from build123d import *
from OCP.BRepFilletAPI import BRepFilletAPI_MakeChamfer

# Parameters (mm, degrees)
SKETCH2_R               = 67.5
SKETCH2_W               = 66.7
SKETCH2_H               = 90
BOSS_EXTRUDE1_DEPTH     = 15
SKETCH7_W               = 14
SKETCH7_H               = 11.1
CUT_EXTRUDE1_DEPTH      = 135.058839694
CUT_EXTRUDE1_DEPTH_BACK = 135.058839694
SKETCH8_R               = 9.5
FILLET1_R               = 20
SKETCH9_R               = 2.1
CUT_EXTRUDE2_DEPTH      = 97.630740606
CHAMFER1_SIZE           = 1.5
CHAMFER1_SIZE2          = 0.866025404
SKETCH10_R              = 4.1
CUT_EXTRUDE3_DEPTH      = 97.630740606
CUT_EXTRUDE4_DEPTH      = 97.630740606
SKETCH12_W              = 10
SKETCH12_H              = 6
CUT_EXTRUDE5_DEPTH      = 97.630740606
CHAMFER2_START          = -1
CHAMFER2_DEPTH          = 16
CUT_EXTRUDE6_DEPTH      = 97.630740606


with BuildPart() as part:
    # Sketch2 → Boss-Extrude1 (new body)
    with BuildSketch(Plane(origin=(0, 0, 0), x_dir=(1, 0, 0), z_dir=(0, 1, 0))):
        with Locations(Location((0, 0, 0), (0, 0, 270))):
            Circle(SKETCH2_R)
        Rectangle(SKETCH2_W, SKETCH2_H, mode=Mode.SUBTRACT)
    extrude(amount=BOSS_EXTRUDE1_DEPTH)

    # Sketch7 → Cut-Revolve2 (revolve, cut)
    with BuildSketch(Plane(origin=(0, 15, 0), x_dir=(1, 0, 0), z_dir=(0, 1, 0))):
        with Locations((-40.35, 5.55)):
            Rectangle(SKETCH7_W, SKETCH7_H)
        with Locations((40.35, 5.55)):
            Rectangle(SKETCH7_W, SKETCH7_H)
    revolve(axis=Axis((67.5, 15, 0), (-1, 0, 0)), mode=Mode.SUBTRACT)

    # Sketch8 → Cut-Extrude1 (cut, two sides: drawn at the far end of the back side and taken through both)
    with BuildSketch(Plane.ZY.offset(-47.35).offset(-CUT_EXTRUDE1_DEPTH_BACK)):
        with Locations((0, 15)):
            Circle(SKETCH8_R)
    extrude(amount=CUT_EXTRUDE1_DEPTH + CUT_EXTRUDE1_DEPTH_BACK, mode=Mode.SUBTRACT)

    # Fillet1
    fillet1_edges = [part.edges().sort_by_distance(p)[0] for p in [
        (-33.35, 7.5, -45),
        (-33.35, 7.5, 45),
        (33.35, 7.5, 45),
        (33.35, 7.5, -45),
    ]]
    fillet(fillet1_edges, radius=FILLET1_R)

    # Sketch9 → Cut-Extrude2 (cut, through all)
    with BuildSketch(Plane(origin=(0, 15, 0), x_dir=(1, 0, 0), z_dir=(0, 1, 0))):
        with Locations(Location((-37.629775444, 17.5, 0), (0, 0, 270))):
            Circle(SKETCH9_R)
        with Locations(Location((37.629775444, 17.5, 0), (0, 0, 270))):
            Circle(SKETCH9_R)
        with Locations(Location((37.629775444, -17.5, 0), (0, 0, 270))):
            Circle(SKETCH9_R)
        with Locations(Location((-37.629775444, -17.5, 0), (0, 0, 270))):
            Circle(SKETCH9_R)
        with Locations(Location((-20, 51.23475383, 0), (0, 0, 270))):
            Circle(SKETCH9_R)
        with Locations(Location((20, 51.23475383, 0), (0, 0, 270))):
            Circle(SKETCH9_R)
        with Locations(Location((20, -51.23475383, 0), (0, 0, 270))):
            Circle(SKETCH9_R)
        with Locations(Location((-20, -51.23475383, 0), (0, 0, 270))):
            Circle(SKETCH9_R)
        with Locations(Location((0, -55, 0), (0, 0, 270))):
            Circle(SKETCH9_R)
        with Locations(Location((0, 58.5, 0), (0, 0, 270))):
            Circle(SKETCH9_R)
        with Locations(Location((-46, 17.5, 0), (0, 0, 270))):
            Circle(SKETCH9_R)
        with Locations(Location((46, 17.5, 0), (0, 0, 270))):
            Circle(SKETCH9_R)
        with Locations(Location((46, -17.5, 0), (0, 0, 270))):
            Circle(SKETCH9_R)
        with Locations(Location((-46, -17.5, 0), (0, 0, 270))):
            Circle(SKETCH9_R)
    extrude(amount=-CUT_EXTRUDE2_DEPTH, mode=Mode.SUBTRACT)

    # Chamfer1: one chamfer whose edges measure the first distance from different faces: ONE call of the kernel's chamfer builder (chamfer() names one face for all edges)
    chamfer1_edges_1 = [part.edges().sort_by_distance(p)[0] for p in [
        (-33.35, 3.9, 0),
    ]]
    chamfer1_side_1 = [part.faces().sort_by_distance(p)[0] for p in [
        (-33.35, 0.522015325, 0),
    ]]
    chamfer1_edges_2 = [part.edges().sort_by_distance(p)[0] for p in [
        (33.35, 3.9, 0),
    ]]
    chamfer1_side_2 = [part.faces().sort_by_distance(p)[0] for p in [
        (33.35, 0.522015325, 0),
    ]]
    chamfer1 = BRepFilletAPI_MakeChamfer(part.part.solid().wrapped)
    for e in chamfer1_edges_1:
        chamfer1.Add(CHAMFER1_SIZE, CHAMFER1_SIZE2, e.wrapped, chamfer1_side_1[0].wrapped)  # the first distance lies on this face
    for e in chamfer1_edges_2:
        chamfer1.Add(CHAMFER1_SIZE, CHAMFER1_SIZE2, e.wrapped, chamfer1_side_2[0].wrapped)  # the first distance lies on this face
    add(Compound.cast(chamfer1.Shape()), mode=Mode.REPLACE)

    # Sketch10 → Cut-Extrude3 (cut, through all)
    with BuildSketch(Plane.XZ):
        with Locations(Location((42.072853481, -42.072853481, 0), (0, 0, 270))):
            Circle(SKETCH10_R)
        with Locations(Location((-42.072853481, -42.072853481, 0), (0, 0, 270))):
            Circle(SKETCH10_R)
        with Locations(Location((-42.072853481, 42.072853481, 0), (0, 0, 270))):
            Circle(SKETCH10_R)
        with Locations(Location((42.072853481, 42.072853481, 0), (0, 0, 270))):
            Circle(SKETCH10_R)
    extrude(amount=-CUT_EXTRUDE3_DEPTH, mode=Mode.SUBTRACT)

    # Sketch11 → Cut-Extrude4 (cut, through all)
    with BuildSketch(Plane.XZ):
        with BuildLine():
            Line((57.5, -35.355339059), (57.5, 35.355339059))
            ThreePointArc((57.5, 35.355339059), (67.5, 0), (57.5, -35.355339059))
        make_face()
    extrude(amount=-CUT_EXTRUDE4_DEPTH, mode=Mode.SUBTRACT)

    # Sketch12 → Cut-Extrude5 (cut, through all)
    with BuildSketch(Plane(origin=(0, 15, 0), x_dir=(1, 0, 0), z_dir=(0, 1, 0))):
        with Locations((0, 48)):
            Rectangle(SKETCH12_W, SKETCH12_H)
    extrude(amount=-CUT_EXTRUDE5_DEPTH, mode=Mode.SUBTRACT)

    # Chamfer2: read off the stored shape, not the designer's step
    # Chamfer2 outline → Chamfer2 (cut)
    with BuildSketch(Plane(origin=(0, 0, 0), x_dir=(1, 0, 0), z_dir=(0, 1, 0)).offset(CHAMFER2_START)):
        with BuildLine():
            Line((14.45, 44.969727089), (8.74275335, 51))
            Line((8.74275335, 51), (5, 51))
            Line((5, 51), (5, 45))
            Line((5, 45), (13.35, 45))
            ThreePointArc((13.35, 45), (13.900208244, 44.99243034), (14.45, 44.969727089))
        make_face()
        with BuildLine():
            Line((-5, 45), (-5, 51))
            Line((-5, 51), (-8.74275335, 51))
            Line((-8.74275335, 51), (-14.45, 44.969727089))
            ThreePointArc((-14.45, 44.969727089), (-13.900208244, 44.99243034), (-13.35, 45))
            Line((-13.35, 45), (-5, 45))
        make_face()
    extrude(amount=CHAMFER2_DEPTH, mode=Mode.SUBTRACT)

    # Sketch13 → Cut-Extrude6 (cut, through all)
    with BuildSketch(Plane.XZ):
        with BuildLine():
            Line((-57.5, -35.355339059), (-57.5, 35.355339059))
            ThreePointArc((-57.5, 35.355339059), (-67.5, 0), (-57.5, -35.355339059))
        make_face()
    extrude(amount=-CUT_EXTRUDE6_DEPTH, mode=Mode.SUBTRACT)


solid = part.part
CAD build for the part. Positions are in the model's coordinates, mm. A direction names the side the tool comes from. Coordinates: 2 decimals unless noted, no trailing zeros. Loops run counter-clockwise (first coordinate to the right, second up) from the corner with the lowest first, then second, coordinate; pieces in that order, holes last. Notation, with made-up numbers: (9.25, -28.5) - (64.25, -28.5) arc R14 cw to (64.25, -22.5) - close; hole circle Ø11 at (32.25, 40.25). An arc over 180 degrees is marked (long way). Write item = value, one per line. Start each with the question number.
Q1. Drill centre lines: L1, parallel to X at y = 6.5, z = 12; L2, parallel to X at y = 1.25, z = 43; L3, parallel to X at y = 3.75, z = -45. Where is each one in solid material? Low to high.
Q2. Cut at C-C, the plane z = 0. List the corners of the cut face in (x, y).
Q3. Cut at A-A, the plane x = 0. List the corners of the cut face in (y, z), then the cut area to 3 significant figures.
Q4. Cut at B-B, the plane z = 17.5. List the corners of the cut face in (x, y).
Q5. Pull direction X, two halves, no side cores. Call faces 3 (the cylindrical face through (0.963, 7.395, -67.493)), 4 (the flat face through (47.35, 5, 0)): pulls with the +X half, pulls with the -X half, needs draft (parallel to the pull), parting line crosses it, or undercut.
Q6. Cut at D-D, the plane y = 11. Give the number of separate pieces and of enclosed holes in the cut face, then the cut area to 3 significant figures.
Q7. Which spindle directions (+Z, -Z, +X, -X, +Y, -Y) get a long thin tool onto all of the face, cutting with end or side? Do faces 1 (the conical face through (34.1, 3.7, -0.2)), 2 (the flat face through (0, 7, 45)). Say none if no direction does.
Q8. Flat gauge pins, fed straight in: pin 1 Ø8 at (x, y) = (-15.5, 5) entering from +Z; pin 2 Ø13 at (x, z) = (42.07, 42.07) entering from -Y; pin 3 Ø2.5 at (x, z) = (20, -51.23) entering from +Y; pin 4 Ø1 at (x, y) = (20.5, 3) entering from +Z. Where does each tip first touch, or does it go through?
Computed:
q1.L1 = -57.5 to -33.35, 33.35 to 57.5
q1.L2 = -52.03 to -46.07, -38.08 to -22.07, 22.07 to 38.08, 46.07 to 52.03
q1.L3 = -50.31 to -44.94, -39.2 to -14.42, 14.42 to 39.2, 44.94 to 50.31
q2.outline = (-57.5, 0) - (-33.35, 0) - (-33.35, 2.4) - (-34.22, 3.9) - (-47.35, 3.9) - (-47.35, 5.5) - (-57.5, 5.5) - close; (33.35, 0) - (57.5, 0) - (57.5, 5.5) - (47.35, 5.5) - (47.35, 3.9) - (34.22, 3.9) - (33.35, 2.4) - close
q3.outline = (0, -67.5) - (15, -67.5) - (15, -60.6) - (0, -60.6) - close; (0, -56.4) - (15, -56.4) - (15, -51) - (0, -51) - close; (0, 45) - (15, 45) - (15, 52.9) - (0, 52.9) - close; (0, 57.1) - (15, 57.1) - (15, 67.5) - (0, 67.5) - close
q3.area = 459 mm²
q4.outline = (-57.5, 0) - (-48.1, 0) - (-48.1, 15) - (-57.5, 15) - close; (-43.9, 0) - (-39.73, 0) - (-39.73, 15) - (-43.9, 15) - close; (-35.53, 0) - (-33.35, 0) - (-33.35, 15) - (-35.53, 15) - close; (33.35, 0) - (35.53, 0) - (35.53, 15) - (33.35, 15) - close; (39.73, 0) - (43.9, 0) - (43.9, 15) - (39.73, 15) - close; (48.1, 0) - (57.5, 0) - (57.5, 15) - (48.1, 15) - close
q5.face_3 = parting line crosses it
q5.face_4 = undercut
q6.separate_pieces = 2
q6.enclosed_holes = 18
q6.area = 6,220 mm²
q7.face_1 = +Y
q7.face_2 = +Y, -Y
q8.pin_1 = 66.51
q8.pin_2 = 0
q8.pin_3 = through
q8.pin_4 = 64.47
